Model file for the job. Use its own axes, mm. Give positions to 0.01 mm unless a question says otherwise; leave off trailing zeros. Write each loop counter-clockwise with the first axis right and the second up, starting at its lowest first coordinate (ties: lowest second). Pieces come first, ordered by that corner, then holes.
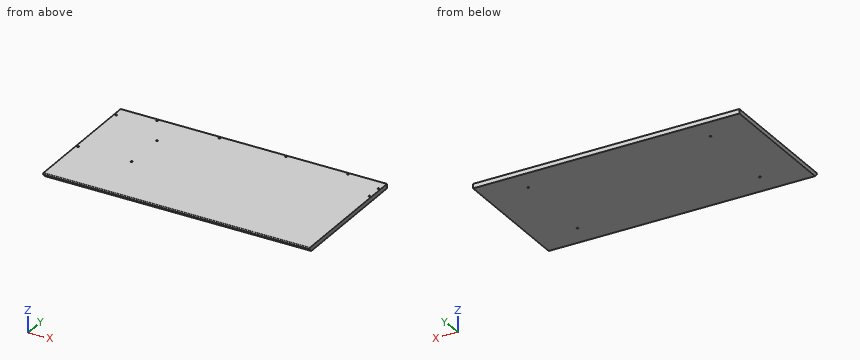
```python
from build123d import *

# Parameters (mm, degrees)
F0_W           = 1200
F0_H           = 600
F1_DEPTH       = 20
F2_R           = 5
F3_SIZE        = 14.99999
F6_D           = 8
F6_DEPTH       = 10
F6_TIP         = 2.4034424761
F6_ON_F5_D     = 8
F6_ON_F5_DEPTH = 10
F6_ON_F5_TIP   = 2.4034424761


# Not quite as in the source:
# - a fillet or chamfer is up to 0.001 mm smaller than in the source, because OpenCascade refuses the exact size


with BuildPart() as f1:
    # F0 (on Top) → F1 (new body)
    with BuildSketch(Plane.XY):
        with Locations((600, -300)):
            Rectangle(F0_W, F0_H)
    extrude(amount=F1_DEPTH)

    # F2
    f2_edges = [f1.edges().sort_by_distance(p)[0] for p in [
        (600, -600, 20),
    ]]
    fillet(f2_edges, radius=F2_R)

    # F3 (size 15 in the source; OpenCascade refuses exactly that, so slightly less here)
    f3_edges = [f1.edges().sort_by_distance(p)[0] for p in [
        (600, -600, 0),
    ]]
    chamfer(f3_edges, length=F3_SIZE)

    # F6
    with Locations(Plane.XY.offset(20)):
        with Locations((1030, -9), (750, -9), (450, -9), (170, -9), (9, -50), (9, -345), (251, -150), (251, -345), (1191, -120), (1191, -50)):
            Hole(F6_D / 2, depth=F6_DEPTH)
            with Locations((0, 0, -(F6_DEPTH + F6_TIP / 2))):  # 118° drill point
                Cone(0, F6_D / 2, F6_TIP, mode=Mode.SUBTRACT)

    # F6 on F5
    with Locations(Plane(origin=(0, 0, 0), x_dir=(1, 0, 0), z_dir=(0, 0, -1))):
        with Locations((189, 482.5), (189, 102.5), (1011, 102.5), (1011, 482.5)):
            Hole(F6_ON_F5_D / 2, depth=F6_ON_F5_DEPTH)
            with Locations((0, 0, -(F6_ON_F5_DEPTH + F6_ON_F5_TIP / 2))):  # 118° drill point
                Cone(0, F6_ON_F5_D / 2, F6_ON_F5_TIP, mode=Mode.SUBTRACT)


solid = f1.part
```
1. Slice it at A-A, the plane z = 4.5. Write the cut outline in (x, y).
Calculated:
outline: (0, -589.5) - (1200, -589.5) - (1200, 0) - (0, 0) - close; hole circle Ø8 at (189, -482.5); hole circle Ø8 at (189, -102.5); hole circle Ø8 at (1011, -482.5); hole circle Ø8 at (1011, -102.5)
2. Pin check, flat tips, straight feed: P1, Ø5, axis at x = 251, y = -150, coming from the +Z side; P2, Ø6.5, axis at x = 1030, y = -9, coming from the +Z side; P3, Ø5, axis at x = 262.5, z = 11, coming from the -Y side. Stop position of each tip, or through.
Calculated:
P1: stops at z = 9.1
P2: stops at z = 9.55
P3: stops at y = -598.5
3. Probe probe 1 along X at (y, z) = (-482.5, 2.25); probe 2 along X at (y, z) = (-9, 16); probe 3 along X at (y, z) = (-50, 14). List the from-to ranges inside material, lowest first.
Calculated:
probe 1: x = 0 to 185, 193 to 1007, 1015 to 1200
probe 2: x = 0 to 166, 174 to 446, 454 to 746, 754 to 1026, 1034 to 1200
probe 3: x = 0 to 5, 13 to 1187, 1195 to 1200
